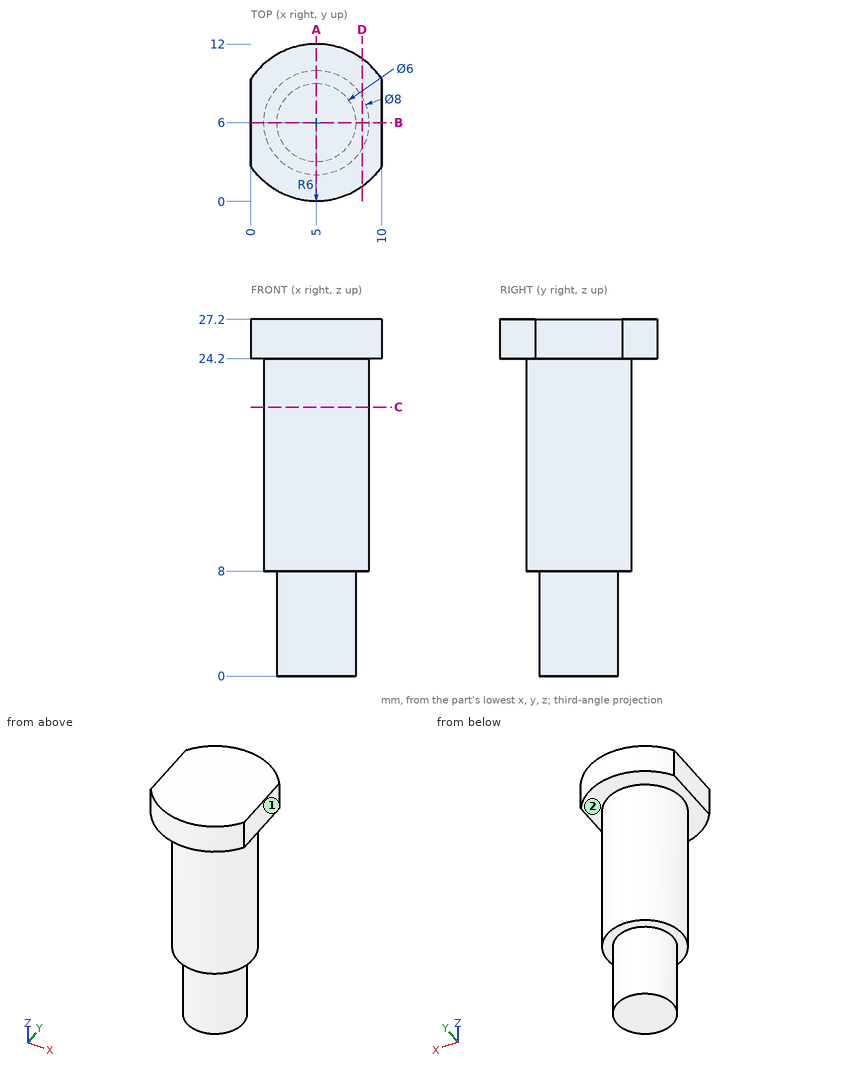
Input: dimensioned drawing with shaded views. Units: mm. Origin: part minimum x, y, z. A direction names the side the tool comes from. Coordinates: 2 decimals unless noted, no trailing zeros. Order: outer loops, then holes, each group sorted by start corner. A loop starts at its lowest first (then second) coordinate and runs counter-clockwise, first axis right, second up. Notation, with made-up numbers: (42.25, 56.5) - (58.25, 56.5) arc R21 cw to (58.25, 84.5) - close; hole circle Ø2 at (22, 0.5). An arc over 180 degrees is marked (long way). Return JSON: item names as keys, results as strings. Group by question number.
1. Cut plane A-A (x = 5). Output: boundary loops of the cut face in (y, z), plus the area to 3 significant figures.
2. Material intervals for line 1 along Z through (x, y) = (3.25, 10.5); line 2 along Z through (x, y) = (6, 3); line 3 along X through (y, z) = (7.5, 10.5), sorted ascending. Write a range as [from, to].
3. Pin query (flat end, axial travel): pin 1 (5 mm diameter, centred on x = 3, z = 13, fed in from -Y); pin 2 (6 mm diameter, centred on y = 6.5, z = 17.5, fed in from +X); pin 3 (3 mm diameter, centred on y = 6.5, z = 21.5, fed in from -X). Return the tip coordinate at first contact, or that it passes through.
4. Set-up query: the marked faces 1 and 2. Return all of +Z, -Z, +X, -X, +Y, -Y with unobstructed straight access to the full face (end or side cutting, diameter ignored); none if empty.
5. Cut plane D-D (x = 8.5). Output: boundary loops of the cut face in (y, z), plus the area to 3 significant figures.
6. Cut plane C-C (z = 20.5). Output: boundary loops of the cut face in (x, y).
7. Cut plane B-B (y = 6). Output: boundary loops of the cut face in (x, z).
Resolved:
{
 "1": {"outline": "(0, 24.2) - (2, 24.2) - (2, 8) - (3, 8) - (3, 0) - (9, 0) - (9, 8) - (10, 8) - (10, 24.2) - (12, 24.2) - (12, 27.2) - (0, 27.2) - close", "area": "214 mm²"},
 "2": {"line 1": "z = [24.2, 27.2]", "line 2": "z = [8, 27.2]", "line 3": "x = [1.29, 8.71]"},
 "3": {"pin 1": "stops at y = 2", "pin 2": "stops at x = 9", "pin 3": "stops at x = 1"},
 "4": {"face 1": "+Z, -Z, +X, +Y, -Y", "face 2": "-Z"},
 "5": {"outline": "(1.13, 24.2) - (4.06, 24.2) - (4.06, 8) - (7.94, 8) - (7.94, 24.2) - (10.87, 24.2) - (10.87, 27.2) - (1.13, 27.2) - close", "area": "92.0 mm²"},
 "6": {"outline": "circle Ø8 at (5, 6)"},
 "7": {"outline": "(0, 24.2) - (1, 24.2) - (1, 8) - (2, 8) - (2, 0) - (8, 0) - (8, 8) - (9, 8) - (9, 24.2) - (10, 24.2) - (10, 27.2) - (0, 27.2) - close"}
}
